```python
from build123d import *

# Parameters (mm, degrees)
SKETCH1_R           = 3.25
SKETCH1_W           = 55.97
SKETCH1_H           = 4
SKETCH1_W_2         = 2
BOSS_EXTRUDE1_DEPTH = 7.5
SKETCH2_R           = 3.25
BOSS_EXTRUDE2_DEPTH = 5
SKETCH3_R           = 1.6
SKETCH3_R_2         = 2.6
CUT_EXTRUDE1_DEPTH  = 10
SKETCH4_R           = 3
SKETCH4_R_2         = 4.5
CUT_EXTRUDE2_DEPTH  = 28.03
BOSS_EXTRUDE3_DEPTH = 12.5
SKETCH6_W           = 59.97
SKETCH6_H           = 32.03
BOSS_EXTRUDE4_DEPTH = 12


with BuildPart() as part:
    # Sketch1 → Boss-Extrude1 (new, symmetric)
    # profile 1 of 8: a face of its own
    with BuildSketch(Plane(origin=(0, 0, 0), x_dir=(1, 0, 0), z_dir=(0, 1, 0))):
        with BuildLine():
            ThreePointArc((24, -0.115), (21.182179477, -1.282179477), (20.015, -4.1))
            Line((20.015, -4.1), (20.015, -10.015))
            Line((20.015, -10.015), (-20.015, -10.015))
            Line((-20.015, -10.015), (-20.015, 10.015))
            Line((-20.015, 10.015), (20.015, 10.015))
            Line((20.015, 10.015), (20.015, 4.1))
            ThreePointArc((20.015, 4.1), (21.182179477, 1.282179477), (24, 0.115))
            ThreePointArc((24, 0.115), (26.817820523, 1.282179477), (27.985, 4.1))
            Line((27.985, 4.1), (27.985, 14.015))
            Line((27.985, 14.015), (-27.985, 14.015))
            Line((-27.985, 14.015), (-27.985, -14.015))
            Line((-27.985, -14.015), (27.985, -14.015))
            Line((27.985, -14.015), (27.985, -4.1))
            ThreePointArc((27.985, -4.1), (26.817820523, -1.282179477), (24, -0.115))
        make_face()
        with Locations(Location((-24, -5, 0), (0, 0, 270))):
            Circle(SKETCH1_R, mode=Mode.SUBTRACT)
        with Locations(Location((24, -5, 0), (0, 0, 270))):
            Circle(SKETCH1_R, mode=Mode.SUBTRACT)
        with Locations(Location((-24, 5, 0), (0, 0, 270))):
            Circle(SKETCH1_R, mode=Mode.SUBTRACT)
        with Locations(Location((24, 5, 0), (0, 0, 270))):
            Circle(SKETCH1_R, mode=Mode.SUBTRACT)
    # profile 2 of 8: a face of its own
    with BuildSketch(Plane(origin=(0, 0, 0), x_dir=(1, 0, 0), z_dir=(0, 1, 0))):
        with Locations((0, -16.015)):
            Rectangle(SKETCH1_W, SKETCH1_H)
    # profile 3 of 8: a face of its own
    with BuildSketch(Plane(origin=(0, 0, 0), x_dir=(1, 0, 0), z_dir=(0, 1, 0))):
        Polygon((27.985, 4.1), (27.985, 0.115), (29.985, 0.115), (29.985, 14.015), (27.985, 14.015), align=None)
    # profile 4 of 8: a face of its own
    with BuildSketch(Plane(origin=(0, 0, 0), x_dir=(1, 0, 0), z_dir=(0, 1, 0))):
        Polygon((29.985, -0.115), (27.985, -0.115), (27.985, -4.1), (27.985, -14.015), (29.985, -14.015), align=None)
    # profile 5 of 8: a face of its own
    with BuildSketch(Plane(origin=(0, 0, 0), x_dir=(1, 0, 0), z_dir=(0, 1, 0))):
        with BuildLine():
            Line((27.985, -4.1), (27.985, -0.115))
            Line((27.985, -0.115), (24, -0.115))
            ThreePointArc((24, -0.115), (26.817820523, -1.282179477), (27.985, -4.1))
        make_face()
    # profile 6 of 8: a face of its own
    with BuildSketch(Plane(origin=(0, 0, 0), x_dir=(1, 0, 0), z_dir=(0, 1, 0))):
        with BuildLine():
            Line((24, 0.115), (27.985, 0.115))
            Line((27.985, 0.115), (27.985, 4.1))
            ThreePointArc((27.985, 4.1), (26.817820523, 1.282179477), (24, 0.115))
        make_face()
    # profile 7 of 8: a face of its own
    with BuildSketch(Plane(origin=(0, 0, 0), x_dir=(1, 0, 0), z_dir=(0, 1, 0))):
        with Locations((28.985, -16.015)):
            Rectangle(SKETCH1_W_2, SKETCH1_H)
    # profile 8 of 8: a face of its own
    with BuildSketch(Plane(origin=(0, 0, 0), x_dir=(1, 0, 0), z_dir=(0, 1, 0))):
        Polygon((-29.985, 14.015), (-29.985, -18.015), (-27.985, -18.015), (-27.985, -14.015), (-27.985, 14.015), align=None)
    extrude(amount=BOSS_EXTRUDE1_DEPTH, both=True)

    # Sketch2 → Boss-Extrude2 (add)
    with BuildSketch(Plane.XZ.offset(7.5)):
        with Locations(Location((24, -5, 0), (0, 0, 90))):
            Circle(SKETCH2_R)
        with Locations(Location((24, 5, 0), (0, 0, 90))):
            Circle(SKETCH2_R)
        with Locations(Location((-24, -5, 0), (0, 0, 90))):
            Circle(SKETCH2_R)
        with Locations(Location((-24, 5, 0), (0, 0, 90))):
            Circle(SKETCH2_R)
    extrude(amount=-BOSS_EXTRUDE2_DEPTH)

    # Sketch3 → Cut-Extrude1 (cut)
    with BuildSketch(Plane.XY.offset(18.015)):
        with Locations((-14.485, 0)):
            Circle(SKETCH3_R)
        with Locations((10.015, 0)):
            Circle(SKETCH3_R_2)
    extrude(amount=-CUT_EXTRUDE1_DEPTH, mode=Mode.SUBTRACT)

    # Sketch4 → Cut-Extrude2 (cut)
    with BuildSketch(Plane(origin=(0, 0, -14.015), x_dir=(-1, 0, 0), z_dir=(0, 0, -1))):
        with Locations((14.485, 0)):
            Circle(SKETCH4_R)
        with Locations((-10.015, 0)):
            Circle(SKETCH4_R_2)
    extrude(amount=-CUT_EXTRUDE2_DEPTH, mode=Mode.SUBTRACT)

    # Sketch5 → Boss-Extrude3 (add)
    with BuildSketch(Plane.XZ.offset(7.5)):
        Polygon((29.985, -4.1), (20.015, -4.1), (20.015, -10.015), (-20.015, -10.015), (-20.015, 10.015), (20.015, 10.015), (20.015, 4.1), (29.985, 4.1), (29.985, 18.015), (-29.985, 18.015), (-29.985, -14.015), (29.985, -14.015), align=None)
    extrude(amount=BOSS_EXTRUDE3_DEPTH)

    # Sketch6 → Boss-Extrude4 (add)
    with BuildSketch(Plane.XZ.offset(20)):
        with Locations((0, 2)):
            Rectangle(SKETCH6_W, SKETCH6_H)
    extrude(amount=BOSS_EXTRUDE4_DEPTH)


solid = part.part
```
Geometry check sheet. Reference: the model listing, model coordinates, mm. A direction names the side the tool comes from. Give positions to 0.01 mm unless a question says otherwise; leave off trailing zeros. Order: outer loops, then holes, each group sorted by start corner. A loop starts at its lowest first (then second) coordinate and runs counter-clockwise, first axis right, second up. Notation, with made-up numbers: (63.5, -38) - (117.5, -38) arc R19 ccw to (117.5, -5) - close; hole circle Ø9 at (65.5, 17.5). An arc over 180 degrees is marked (long way). Write item = value, one per line. Start each with the question number.
1) Section check B-B (z = -11). Enter the section's corners in (x, y) (3 decimals).
2) Scan lines: L1, parallel to Z at x = -24, y = 2.75 (3 decimals); L2, parallel to Z at x = 5, y = -5 (3 decimals); L3, parallel to X at y = -4, z = 5.5 (3 decimals). Record each from-to range of solid material in increasing order.
3) Section check A-A (x = -24). Enter the section's corners in (y, z) (3 decimals).
4) Access from +Z, -Z, +X, -X, +Y, -Y to the whole of each face (thin tool, end or side, straight path). Record for faces 4 (the flat face through (0, 7.5, 12)), 5 (the flat face through (27, 0, 0.115)), 6 (the flat face through (25, -14, -4.1)), 7 (the flat face through (24, -2.5, 5)), 8 (the cylindrical face through (-11.488, 0.132, 11.987)).
5) Draft check along X on faces 1 (the flat face through (-29.985, -12, 2)), 2 (the flat face through (0, -12, -14.015)), 3 (the flat face through (-20.015, -6, 0)). Enter one of: released by +X, released by -X, zero draft, split by the parting line, or undercut.
6) Section check C-C (y = 0). Count the separate pieces of the cut face and the enclosed holes in it, then the cut area to 3 significant figures.
7) Section check D-D (x = -14.5). Enter the section's corners in (y, z) (3 decimals), then the cut area to 3 significant figures.
8) Gauge pin test, flat end, axial feed: pin 1 Ø2 at (x, z) = (-23, -4) entering from +Y. Record the tip position at first contact, or that the pin passes through.
Geometry check:
q1.outline = (-29.985, -32) - (29.985, -32) - (29.985, 7.5) - (-29.985, 7.5) - close; hole circle Ø6 at (-14.485, 0); hole circle Ø9 at (10.015, 0)
q2.L1 = -14.015 to -8.25, -1.75 to 1.75, 8.25 to 18.015
q2.L2 = -14.015 to -10.015, 10.015 to 18.015
q2.L3 = -29.985 to -20.015, 20.015 to 29.985
q3.outline = (-32, -14.015) - (7.5, -14.015) - (7.5, -8.25) - (-2.5, -8.25) - (-2.5, -1.75) - (7.5, -1.75) - (7.5, 1.75) - (-2.5, 1.75) - (-2.5, 8.25) - (7.5, 8.25) - (7.5, 18.015) - (-32, 18.015) - close
q4.face_4 = +Z, -Z, +X, -X, +Y
q4.face_5 = +X, +Y
q4.face_6 = +X
q4.face_7 = +Y
q4.face_8 = -Z
q5.face_1 = released by -X
q5.face_2 = zero draft
q5.face_3 = undercut
q6.separate_pieces = 5
q6.enclosed_holes = 4
q6.area = 824 mm2
q7.outline = (-32, -14.015) - (-3, -14.015) - (-3, -10.015) - (-20, -10.015) - (-20, 10.015) - (-3, 10.015) - (-3, 14.015) - (-1.6, 14.015) - (-1.6, 18.015) - (-32, 18.015) - close; (1.6, 14.015) - (3, 14.015) - (3, 10.015) - (7.5, 10.015) - (7.5, 18.015) - (1.6, 18.015) - close; (3, -14.015) - (7.5, -14.015) - (7.5, -10.015) - (3, -10.015) - close
q7.area = 654 mm2
q8.pin_1 = -2.5
